Build history of the part. All positions in model axes, mm. Face numbers are marked on the shaded views. A direction names the side the tool comes from. Give positions to 0.01 mm unless a question says otherwise; leave off trailing zeros. Write each loop counter-clockwise with the first axis right and the second up, starting at its lowest first coordinate (ties: lowest second). Pieces come first, ordered by that corner, then holes. Notation, with made-up numbers: (-37, 65.25) -> (-30, 65.25) arc R22 cw to (-30, 91.25) -> close; hole circle Ø5 at (65.5, -9). An arc over 180 degrees is marked (long way). Put each result on its own line as item: value. Start each with the question number.
Item 1: Flat gauge pins, fed straight in: pin 1 Ø2 at (x, z) = (-20, 4) entering from -Y; pin 2 Ø2 at (x, z) = (-43, 17) entering from -Y; pin 3 Ø1 at (x, z) = (-36, 6) entering from -Y; pin 4 Ø4 at (x, y) = (-27.5, -9) entering from -Z. Where does each tip first touch, or does it go through?
Item 2: Drill centre lines: line 1 along X through (y, z) = (-2, 20.5); line 2 along Y through (x, z) = (-64.5, -9.5); line 3 along Y through (x, z) = (-51.5, 2). Where is each one in solid material? Low to high.
Item 3: Slice it at D-D, the plane x = -62. List the corners of the cut face in (y, z).
Item 4: Slice it at A-A, the plane z = 0. List the corners of the cut face in (x, y).
Item 5: Tool access for the marked faces 1, 2 and 3: list every direction of +Z, -Z, +X, -X, +Y, -Y with a clear straight run to the whole face (end or side of a thin tool).
Item 6: Slice it at C-C, the plane x = -30.5. List the corners of the cut face in (y, z), plus the area to 3 significant figures.
```python
from build123d import *

# Parameters (mm, degrees)
CHANFREIN1_SIZE = 1
CHANFREIN2_SIZE = 3


with BuildPart() as part:
    # Esquisse1 → Révolution1 (revolve)
    with BuildSketch(Plane.XY, mode=Mode.PRIVATE) as r_volution1_sk:
        Polygon((0, 0), (0, 15), (-8, 15), (-8, 22.5), (-22.5, 22.5), (-22.5, 15), (-42.5, 15), (-79.5, 12.5), (-102.5, 12.5), (-102.5, 11.9), (-103.8, 11.9), (-103.8, 12.5), (-107.5, 12.5), (-107.5, 0), align=None)
    revolve(r_volution1_sk.sketch.rotate(Axis((0, 0, 0), (-1, 0, 0)), 90), axis=Axis((0, 0, 0), (-1, 0, 0)))  # turned: the seam where the file's is

    # Chanfrein1
    chanfrein1_edges = [part.edges().sort_by_distance(p)[0] for p in [
        (-107.5, 0, 12.5),
    ]]
    chamfer(chanfrein1_edges, length=CHANFREIN1_SIZE)

    # Chanfrein2
    chanfrein2_edges = [part.edges().sort_by_distance(p)[0] for p in [
        (0, 0, 15),
    ]]
    chamfer(chanfrein2_edges, length=CHANFREIN2_SIZE)


solid = part.part
```
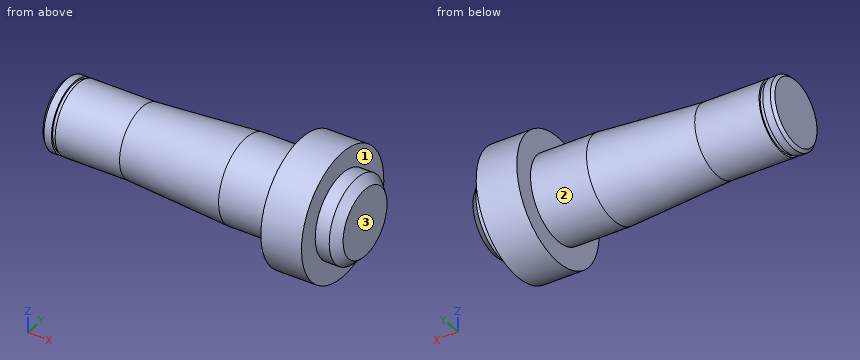
Values follow:
1. pin 1: y = -22.3
1. pin 2: through
1. pin 3: y = -13.96
1. pin 4: z = -13.27
2. line 1: -22.5 to -8
2. line 2: -9.61 to 9.61
2. line 3: -14.25 to 14.25
3. outline: circle Ø27.36 at (0, 0)
4. outline: (-107.5, -11.5) -> (-106.5, -12.5) -> (-103.8, -12.5) -> (-103.8, -11.9) -> (-102.5, -11.9) -> (-102.5, -12.5) -> (-79.5, -12.5) -> (-42.5, -15) -> (-22.5, -15) -> (-22.5, -22.5) -> (-8, -22.5) -> (-8, -15) -> (-3, -15) -> (0, -12) -> (0, 12) -> (-3, 15) -> (-8, 15) -> (-8, 22.5) -> (-22.5, 22.5) -> (-22.5, 15) -> (-42.5, 15) -> (-79.5, 12.5) -> (-102.5, 12.5) -> (-102.5, 11.9) -> (-103.8, 11.9) -> (-103.8, 12.5) -> (-106.5, 12.5) -> (-107.5, 11.5) -> close
5. face 1: +X
5. face 2: -X
5. face 3: +Z, -Z, +X, +Y, -Y
6. outline: circle Ø30 at (0, 0)
6. area: 707 mm2
